Geometry: see drawing. Coordinates: mm, zero at the bounding-box minimum. A direction names the side the tool comes from. Coordinates: 2 decimals unless noted, no trailing zeros. Loops run counter-clockwise (first coordinate to the right, second up) from the corner with the lowest first, then second, coordinate; pieces in that order, holes last. Notation, with made-up numbers: (-23.75, 16) - (33.25, 16) arc R20 ccw to (33.25, 40) - close; hole circle Ø9 at (58.25, -8). An arc over 180 degrees is marked (long way). Use a Markdown table: item, result. Add a question column.
1. Section query A-A on z = 9.5. Return the cut outline in (x, y), then the cut area to 4 significant figures.
2. Section query C-C on x = 23.5. Return the cut outline in (y, z).
3. Section query D-D on z = 17.5. State how many separate pieces and enclosed holes the cut face has, then the cut area to 3 significant figures.
4. Ray query, L1, parallel to Z at x = 23.5, y = 0.5; L2, parallel to Z at x = 15, y = 14.75; L3, parallel to X at y = 6.75, z = 17. Return the intervals inside material, ascending. Write a range as [from, to].
5. Contact query for flat-ended pins moving along their axis: P1, Ø4, axis at x = 13.5, z = 22, coming from the +Y side; P2, Ø2.5, axis at y = 15, z = 17.5, coming from the -X side; P3, Ø5.5, axis at x = 38.5, z = 17, coming from the -Y side. Output: stop coordinate, or through.
6. Access query for the marked faces 1, 2 and 3. Directions: +Z, -Z, +X, -X, +Y, -Y. A direction counts if a zero-diameter tool reaches every point of the face in a straight line with its end or side. Return the directions, or none.
7. Section query B-B on y = 15. Return the cut outline in (x, z).
8. Draft query along X for the marked faces 4, 5 and 6. Return one class per face: released by +X, released by -X, zero draft, split by the parting line, or undercut.
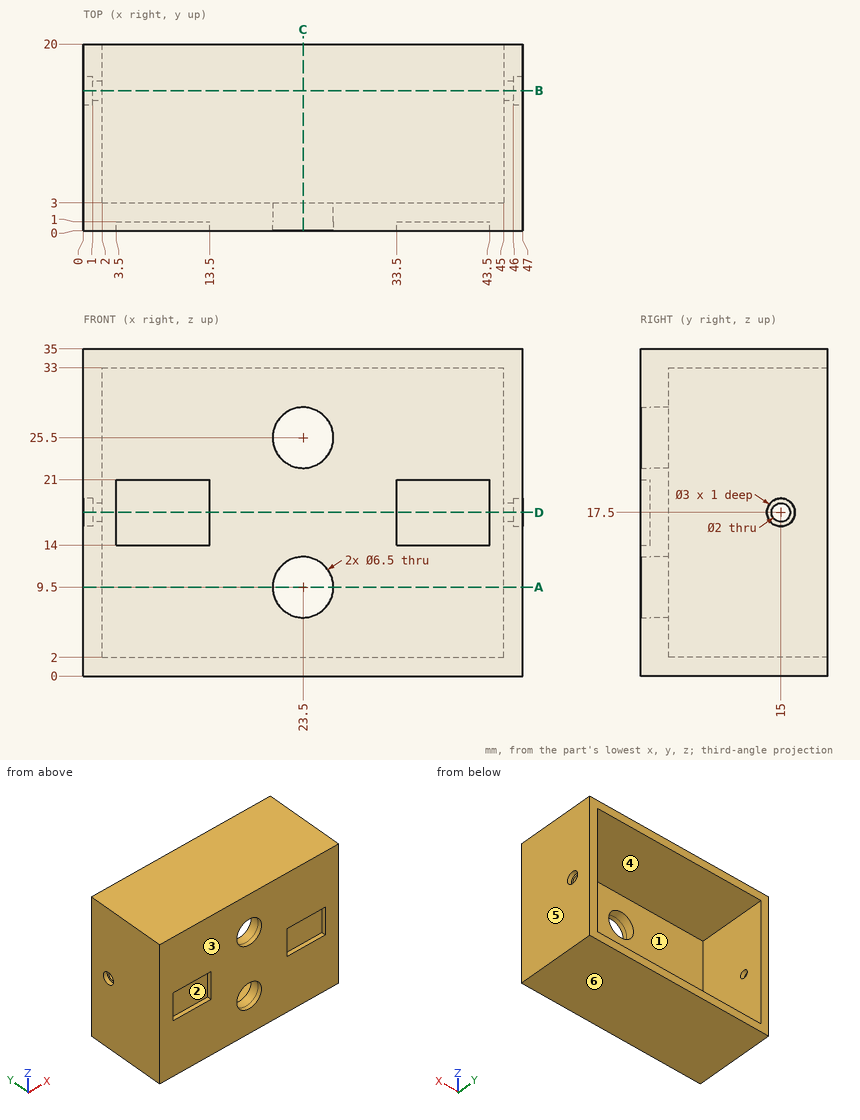
Resolved:
| question | item | result |
|---|---|---|
| 1 | outline | (0, 0) - (20.25, 0) - (20.25, 3) - (2, 3) - (2, 20) - (0, 20) - close; (26.75, 0) - (47, 0) - (47, 20) - (45, 20) - (45, 3) - (26.75, 3) - close |
| 1 | area | 189.5 mm² |
| 2 | outline | (0, 0) - (20, 0) - (20, 2) - (3, 2) - (3, 6.25) - (0, 6.25) - close; (0, 12.75) - (3, 12.75) - (3, 22.25) - (0, 22.25) - close; (0, 28.75) - (3, 28.75) - (3, 33) - (20, 33) - (20, 35) - (0, 35) - close |
| 3 | separate pieces | 3 |
| 3 | enclosed holes | 0 |
| 3 | area | 179 mm² |
| 4 | L1 | [0, 6.25], [12.75, 22.25], [28.75, 35] |
| 4 | L2 | [0, 2], [33, 35] |
| 4 | L3 | [0, 2], [45, 47] |
| 5 | P1 | y = 3 |
| 5 | P2 | x = 1 |
| 5 | P3 | y = 1 |
| 6 | face 1 | +Y |
| 6 | face 2 | -Y |
| 6 | face 3 | +Z, -Z, +X, -X, -Y |
| 7 | outline | (0, 0) - (47, 0) - (47, 16) - (46, 16) - (46, 16.5) - (45, 16.5) - (45, 2) - (2, 2) - (2, 16.5) - (1, 16.5) - (1, 16) - (0, 16) - close; (0, 19) - (1, 19) - (1, 18.5) - (2, 18.5) - (2, 33) - (45, 33) - (45, 18.5) - (46, 18.5) - (46, 19) - (47, 19) - (47, 35) - (0, 35) - close |
| 8 | face 4 | undercut |
| 8 | face 5 | released by +X |
| 8 | face 6 | zero draft |
